Print and shaded views of the part. All mm, measured from the part's lowest x, y and z. A direction names the side the tool comes from. Give positions to 0.01 mm unless a question says otherwise; leave off trailing zeros. Loops run counter-clockwise (first coordinate to the right, second up) from the corner with the lowest first, then second, coordinate; pieces in that order, holes last. Notation, with made-up numbers: M 50.5,0 L 69.5,0 A25 cw 69.5,26 Z; hole C 23.25,59.5 d10. An arc over 180 degrees is marked long. Answer in a Markdown table with one row per item.
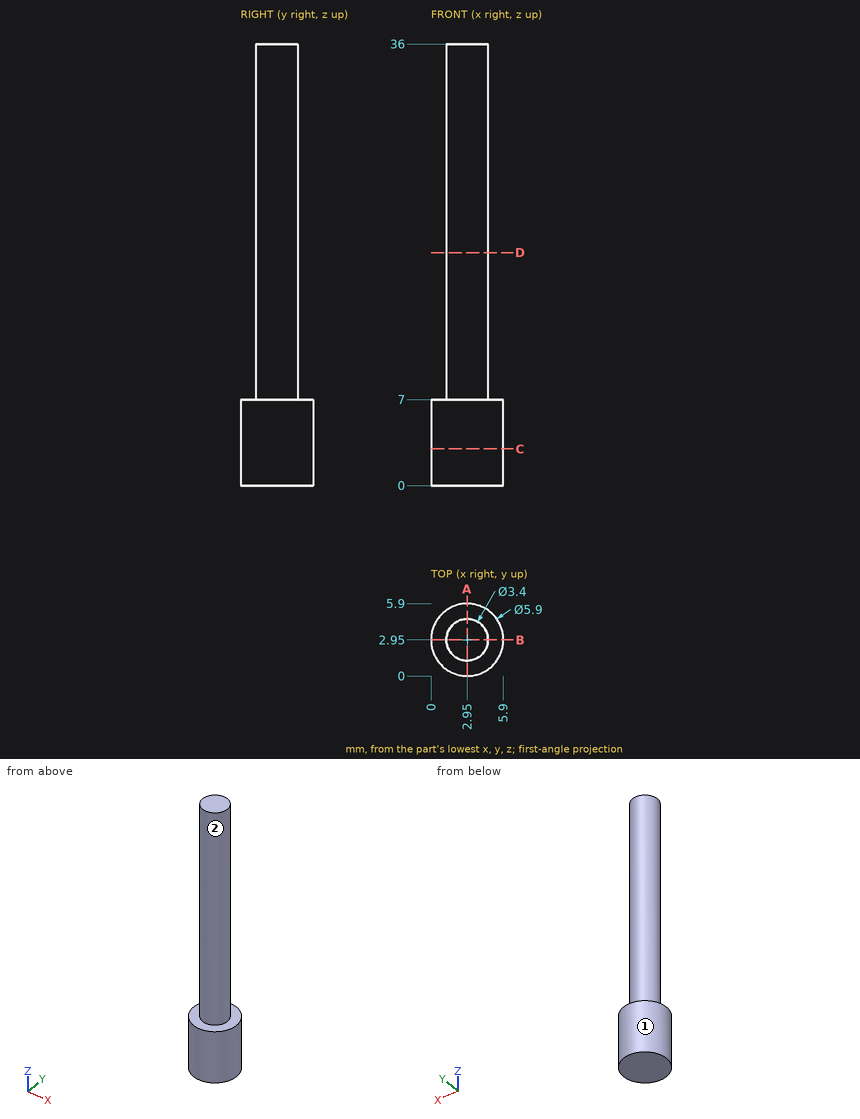
(1) Which spindle directions (+Z, -Z, +X, -X, +Y, -Y) get a long thin tool onto all of the face, cutting with end or side? Do the marked faces 1 and 2. Say none if no direction does.
Established:
| item | result |
|---|---|
| face 1 | +Z, -Z |
| face 2 | +Z |
(2) Saw through at D-D, the plane z = 19. Give the cut face in (x, y), and give its area (3 significant figures).
Established:
| item | result |
|---|---|
| outline | C 2.95,2.95 d3.4 |
| area | 9.08 mm2 |
(3) Flat gauge pins, fed straight in: P1, Ø1, axis at x = 3.5, y = 0.5, coming from the -Z side; P2, Ø2, axis at x = 2.5, z = 24.5, coming from the -Y side. Where does each tip first touch, or does it go through?
Established:
| item | result |
|---|---|
| P1 | stops at z = 0 |
| P2 | stops at y = 1.25 |
(4) Wall check: L1, parallel to X at y = 3.1, z = 2.5; L2, parallel to Z at x = 0.4, y = 3.5. Give the ranges that are in metal, low to high.
Established:
| item | result |
|---|---|
| L1 | x = 0 to 5.9 |
| L2 | z = 0 to 7 |
(5) Saw through at A-A, the plane x = 2.95. Give the cut face in (y, z), and give its area (3 significant figures).
Established:
| item | result |
|---|---|
| outline | M 0,0 L 5.9,0 L 5.9,7 L 4.65,7 L 4.65,36 L 1.25,36 L 1.25,7 L 0,7 Z |
| area | 140 mm2 |
(6) Saw through at C-C, the plane z = 3. Give the cut face in (x, y), and give its area (3 significant figures).
Established:
| item | result |
|---|---|
| outline | C 2.95,2.95 d5.9 |
| area | 27.3 mm2 |
